```python
from build123d import *

# Parameters (mm, degrees)
F1_DEPTH = 0.5715
F2_DEPTH = 0.5715
F4_DEPTH = 5.6444444445


with BuildPart() as f1:
    # F0 (on Front) → F1 (new body)
    with BuildSketch(Plane.XZ):
        with BuildLine():
            ThreePointArc((12.7, 0), (9.3803824016, 15.5542598667), (0, 28.3980633142))
            Line((0, 28.3980633142), (0, -28.3980633142))
            ThreePointArc((0, -28.3980633142), (9.3803824016, -15.5542598667), (12.7, 0))
        make_face()
        with BuildLine():
            Line((0, -28.3980633142), (0, 28.3980633142))
            ThreePointArc((0, 28.3980633142), (-12.7, 0), (0, -28.3980633142))
        make_face()
        with BuildLine():
            ThreePointArc((63.5, 0), (40.9542598667, 34.7803824016), (0, 28.3980633142))
            ThreePointArc((0, 28.3980633142), (9.3803824016, 15.5542598667), (12.7, 0))
            ThreePointArc((12.7, 0), (9.3803824016, -15.5542598667), (0, -28.3980633142))
            ThreePointArc((0, -28.3980633142), (40.9542598667, -34.7803824016), (63.5, 0))
        make_face()
        with BuildLine():
            ThreePointArc((0, -28.3980633142), (-12.7, 0), (0, 28.3980633142))
            ThreePointArc((0, 28.3980633142), (-63.5, 0), (0, -28.3980633142))
        make_face()
    extrude(amount=F1_DEPTH)

    # F2 (add): a face of the model
    f2_faces = [f1.faces().sort_by_distance(p)[0] for p in [
        (0, 0, 0),
    ]]
    extrude(f2_faces, amount=F2_DEPTH)

    # F3 (on face) → F4 (join)
    with BuildSketch(Plane.XZ.offset(0.5715)):
        with BuildLine():
            ThreePointArc((0, -19.05), (4.7206947131, -10.040231571), (6.35, 0))
            ThreePointArc((6.35, 0), (4.7206947131, 10.040231571), (0, 19.05))
            ThreePointArc((0, 19.05), (-6.35, 0), (0, -19.05))
        make_face()
        with BuildLine():
            ThreePointArc((0, 19.05), (4.7206947131, 10.040231571), (6.35, 0))
            ThreePointArc((6.35, 0), (4.7206947131, -10.040231571), (0, -19.05))
            ThreePointArc((0, -19.05), (35.440231571, -30.1206947131), (57.15, 0))
            ThreePointArc((57.15, 0), (35.440231571, 30.1206947131), (0, 19.05))
        make_face()
        with BuildLine():
            ThreePointArc((0, -19.05), (-6.35, 0), (0, 19.05))
            ThreePointArc((0, 19.05), (-57.15, 0), (0, -19.05))
        make_face()
    extrude(amount=F4_DEPTH)


solid = f1.part
```
Verification items for the finished model (mm, model axes). A direction names the side the tool comes from. Round coordinates to 2 decimals unless told otherwise and drop trailing zeros. Order: outer loops, then holes, each group sorted by start corner. A loop starts at its lowest first (then second) coordinate and runs counter-clockwise, first axis right, second up. Notation, with made-up numbers: (45.25, 47) -> (50.25, 47) arc R33 cw to (50.25, 80) -> close; hole circle Ø4 at (50.25, -22). An arc over 180 degrees is marked (long way). Put each result on its own line as item: value. Start each with the question number.
(1) Tool access check on faces 3 (the face through (-63.48, -0.01, 1.23)), 4 (the face through (0, -0.572, 20)). Record the directions out of +Z, -Z, +X, -X, +Y, -Y that give a thin tool (end or side, any length) a straight path to the whole face; none if there is none.
(2) Section check A-A (x = 25.4). Enter the section's corners in (y, z).
(3) Depth check by flat-ended pin: pin 1 Ø2 at (x, y) = (25.5, -3.5) entering from -Z; pin 2 Ø1.5 at (y, z) = (-3, 2.5) entering from -X. Enter the tip coordinate at first touch or a pass-through.
(4) Draft check along X on faces 1 (the face through (-1, 0.572, 1)), 2 (the face through (63.48, -0.01, -1.23)). Enter one of: +X half, -X half, draft (parallel to the pull), parting line (faces both ways), or undercut.
(5) Section check C-C (y = -3.25). Enter the section's corners in (x, z).
(6) Section check B-B (z = -6). Enter the section's corners in (x, y).
(7) Material ranges on line 1 along X through (y, z) = (-4.25, 29); line 2 along X through (y, z) = (-4.5, -21.5); line 3 along Y through (x, z) = (2, 23.5), recorded low to high.
Completed:
1. face 3: +Y, -Y
1. face 4: -Y
2. outline: (-6.22, -31.75) -> (-0.57, -31.75) -> (-0.57, -38.1) -> (0.57, -38.1) -> (0.57, 38.1) -> (-0.57, 38.1) -> (-0.57, 31.75) -> (-6.22, 31.75) -> close
3. pin 1: stops at z = -31.75
3. pin 2: stops at x = -57.1
4. face 1: draft
4. face 2: undercut
5. outline: (0, -19.05) arc R31.75 ccw (long way) to (0, 19.05) arc R31.75 ccw (long way) to start
6. outline: (-63.02, -0.57) -> (-56.58, -0.57) -> (-56.58, -6.22) -> (56.58, -6.22) -> (56.58, -0.57) -> (63.02, -0.57) -> (63.02, 0.57) -> (-63.02, 0.57) -> close
7. line 1: x = -38.33 to -12.47, 12.47 to 38.33
7. line 2: x = -48.76 to -2.04, 2.04 to 48.76
7. line 3: y = -0.57 to 0.57
